Print and shaded views of the part. All mm, measured from the part's lowest x, y and z. Give positions to 0.01 mm unless a question says otherwise; leave off trailing zeros. Loops run counter-clockwise (first coordinate to the right, second up) from the corner with the lowest first, then second, coordinate; pieces in that order, holes last.
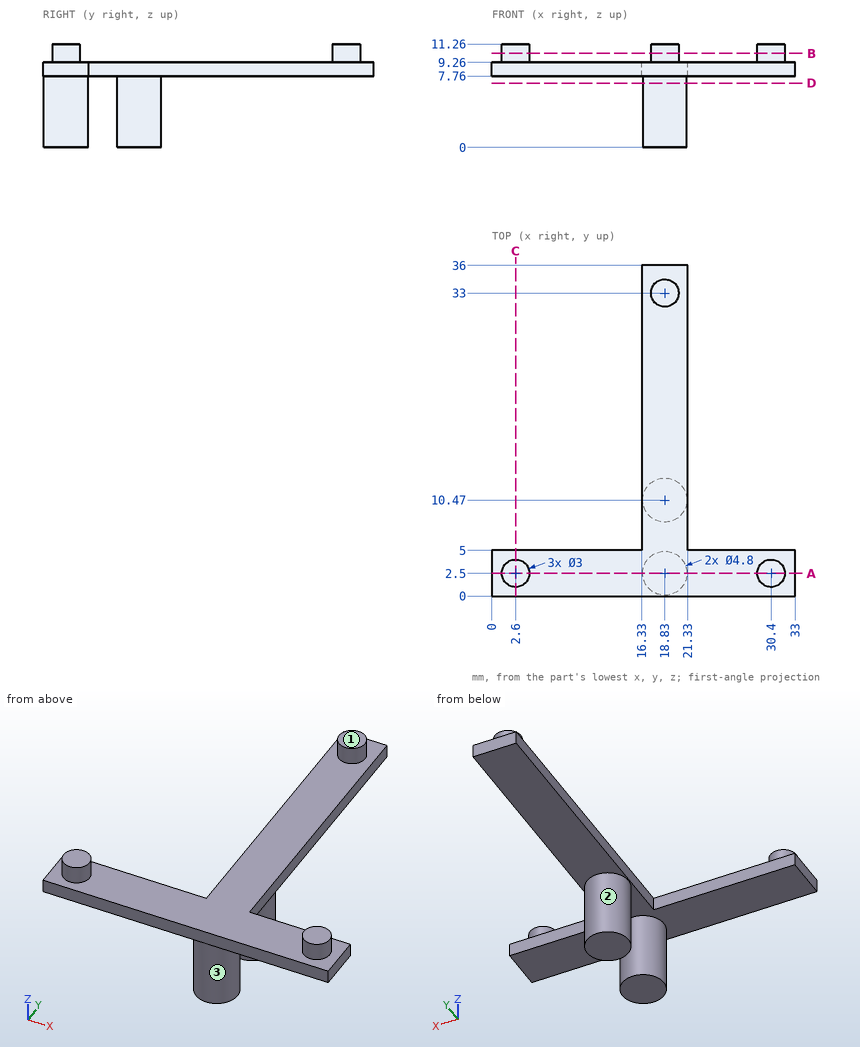
1. Saw through at D-D, the plane z = 7. List the corners of the cut face in (x, y), and give its area (3 significant figures).
Responses:
outline: circle Ø4.8 at (18.83, 2.5); circle Ø4.8 at (18.83, 10.47)
area: 36.2 mm2
2. Saw through at A-A, the plane y = 2.5. List the corners of the cut face in (x, z).
Responses:
outline: (0, 7.76) - (16.43, 7.76) - (16.43, 0) - (21.23, 0) - (21.23, 7.76) - (33, 7.76) - (33, 9.26) - (31.9, 9.26) - (31.9, 11.26) - (28.9, 11.26) - (28.9, 9.26) - (4.1, 9.26) - (4.1, 11.26) - (1.1, 11.26) - (1.1, 9.26) - (0, 9.26) - close
3. Drop flat-ended pins along their axis: pin 1 (4 mm diameter, centred on y = 24.5, z = 6.5, fed in from +X); pin 2 (1.5 mm diameter, centred on x = 17, z = 3, fed in from +Y); pin 3 (0.8 mm diameter, centred on y = 18, z = 9, fed in from -X); pin 4 (10 mm diameter, centred on x = 9.5, y = 30.5, fed in from -Z). Give the stop position or say it passes through.
Responses:
pin 1: stops at x = 21.33
pin 2: stops at y = 12.61
pin 3: stops at x = 16.33
pin 4: passes through
4. Probe line 1 along Y through (x, z) = (19, 7.5); line 2 along Y through (x, z) = (3.5, 8); line 3 along Z through (x, y) = (11.5, 3.5). List the from-to ranges inside material, lowest first.
Responses:
line 1: y = 0.11 to 4.89, 8.08 to 12.86
line 2: y = 0 to 5
line 3: z = 7.76 to 9.26
5. Pull direction Y, two halves, no side cores. Call the marked faces 1, 2 and 3: released by +Y, released by -Y, zero draft, split by the parting line, or undercut.
Responses:
face 1: zero draft
face 2: undercut
face 3: undercut
6. Saw through at C-C, the plane x = 2.6. List the corners of the cut face in (y, z).
Responses:
outline: (0, 7.76) - (5, 7.76) - (5, 9.26) - (4, 9.26) - (4, 11.26) - (1, 11.26) - (1, 9.26) - (0, 9.26) - close
7. Saw through at B-B, the plane z = 10.25. List the corners of the cut face in (x, y).
Responses:
outline: circle Ø3 at (2.6, 2.5); circle Ø3 at (18.83, 33); circle Ø3 at (30.4, 2.5)
